The model under review builds one solid part; all positions refer to its coordinate system, in mm. A direction names the side the tool comes from. Coordinates: 2 decimals unless noted, no trailing zeros. Loops run counter-clockwise (first coordinate to the right, second up) from the corner with the lowest first, then second, coordinate; pieces in that order, holes last. Notation, with made-up numbers: M -6.75,14 L 14.25,14 A6 cw 14.25,24 Z; hole C 63.5,-10.5 d6. An arc over 180 degrees is marked long. Write item = value, one per line. Start each with the question number.
Q1. We need section A-A on y = -65.5. Give the boundary of the cut face in (x, z).
Q2. We need section B-B on y = -111. Give the boundary of the cut face in (x, z), and give its area (3 significant figures).
Q3. We need section C-C on z = -3. Count the separate pieces of the cut face and the enclosed holes in it, and give its area (3 significant figures).
Q4. Clearance check with flat-ended pins moving along their axes: pin 1 Ø20 at (y, z) = (-164.5, 1) entering from -X; pin 2 Ø8 at (x, y) = (-12.5, 2.5) entering from +Z; pin 3 Ø5 at (x, y) = (2, -159.5) entering from +Z; pin 4 Ø15 at (x, y) = (-103.97, -30.81) entering from -Z. State where each tip first meets the part, or that it passes through.
Q5. We need section D-D on y = -163. Give the boundary of the cut face in (x, z), and give its area (3 significant figures).
Q6. Wall thickness on probe 1 along Y at (x, z) = (-36, 3.5); probe 2 along Y at (x, z) = (2, 33); probe 3 along Z at (x, y) = (21, -170): over which ranges is each line inside the solid? List them lowest first.
Q7. For faces 1 (the face through (-17.63, 43.38, -5.55)), 2 (the face through (-84.874, 4.13, 0.21)), 3 (the face through (-28.622, -66.375, -9.014)), list the 3-axis set-ups (+Z, -Z, +X, -X, +Y, -Y) from which the entire face can be reached by the end or side of a thin tool; tool diameter is ignored.
Q8. Mouldability with a two-part tool opening along X and no side actions: class faces 4 (the face through (-120.508, -137.418, 0.21)), 5 (the face through (45.486, -200.478, -1.704)), 6 (the face through (-64.24, -171.38, -0.21)) as released by +X, released by -X, zero draft, split by the parting line, or undercut.
from build123d import *

# Parameters (mm, degrees)
BOSS_EXTRUDE1_DEPTH      = 15
BOSS_EXTRUDE1_DEPTH_BACK = 15
SKETCH3_R                = 12.5
SKETCH4_R                = 30
SKETCH4_R_2              = 25
BOSS_EXTRUDE2_DEPTH      = 60
BOSS_EXTRUDE3_DEPTH      = 5
BOSS_EXTRUDE3_DEPTH_BACK = 25
SKETCH5_R                = 30
FILLET1_R                = 10
CUT_EXTRUDE1_START       = -65
SKETCH6_R                = 25
CUT_EXTRUDE1_DEPTH       = 65


with BuildPart() as part:
    # Sketch2 → Revolve1 (revolve)
    with BuildSketch(Plane.XY, mode=Mode.PRIVATE) as revolve1_sk:
        Polygon((0, 47.481515712), (18.484288355, 47.481515712), (18.484288355, 39.394639556), (44.872104392, 39.394639556), (44.872104392, 24.346445364), (35.445928293, 24.346445364), (35.445928293, -47.074965844), (30.007749775, -47.074965844), (30.007749775, -85.142215473), (18.546286043, -160.936690765), (18.546286043, -189.740958038), (45.517560074, -189.740958038), (45.517560074, -202.518484288), (0, -202.518484288), align=None)
    revolve(revolve1_sk.sketch.rotate(Axis((0, 47.481515712, 0), (0, -1, 0)), 180), axis=Axis((0, 47.481515712, 0), (0, -1, 0)))

    # Sketch3 → Boss-Extrude1 (add, two sides: drawn at the far end of the back side and taken through both)
    with BuildSketch(Plane.XY.offset(-BOSS_EXTRUDE1_DEPTH_BACK)):
        Polygon((-42.28533841, 24.346445364), (-86.474429819, 5.279737536), (-86.474429819, -152.790196511), (-42.28533841, -189.740958038), (-42.28533841, -202.518484288), (-44.080740722, -202.518484288), (-121.474429819, -137.802155929), (-121.474429819, 5.226132785), (-42.28533841, 39.394639556), align=None)
        with Locations((-103.974429819, -30.80530006)):
            Circle(SKETCH3_R, mode=Mode.SUBTRACT)
        with Locations((-103.974429819, -115.80530006)):
            Circle(SKETCH3_R, mode=Mode.SUBTRACT)
    extrude(amount=BOSS_EXTRUDE1_DEPTH + BOSS_EXTRUDE1_DEPTH_BACK)

    # Sketch4 → Boss-Extrude2 (add)
    with BuildSketch(Plane(origin=(0, 0, 0), x_dir=(0, 0, -1), z_dir=(1, 0, 0))):
        with Locations(Location((0, -170, 0), (0, 0, 221.149949101))):
            Circle(SKETCH4_R)
        with Locations(Location((0, -170, 0), (0, 0, 141.388518695))):
            Circle(SKETCH4_R_2, mode=Mode.SUBTRACT)
    extrude(amount=BOSS_EXTRUDE2_DEPTH)

    # Sketch5 → Boss-Extrude3 (add, two sides: drawn at the far end of the back side and taken through both)
    with BuildSketch(Plane(origin=(0, 0, 0), x_dir=(0, 0, -1), z_dir=(1, 0, 0)).offset(-BOSS_EXTRUDE3_DEPTH_BACK)):
        with Locations(Location((0, -170, 0), (0, 0, 221.149949101))):
            Circle(SKETCH5_R)
    extrude(amount=BOSS_EXTRUDE3_DEPTH + BOSS_EXTRUDE3_DEPTH_BACK)

    # Fillet1
    # the kernel refuses this fillet: 10 mm, written as the material it adds along each edge
    with BuildSketch(Plane(origin=(-42.974972659, -189.740958038, 15), x_dir=(-1, 0, 0), z_dir=(0, -1, 0))) as fillet1_piece_1_section:
        with BuildLine():
            CenterArc((6.59517437, -10), FILLET1_R, 90, 63.23655504)
            ThreePointArc((-2.333558622, -5.49692026), (-1.076535169, -2.786770672), (0, 0))
            Line((0, 0), (6.59517437, 0))
        make_face()
    fillet1_piece_1 = extrude(amount=12.777526251, mode=Mode.PRIVATE)
    fillet1_piece_1 = split(fillet1_piece_1, bisect_by=Plane(origin=(-48.522573574, -198.80423941, 19.040168561), z_dir=(0.6414797327096047, 0.7671399823518614, 0)), keep=Keep.TOP, mode=Mode.PRIVATE)
    add(fillet1_piece_1)
    with BuildSketch(Plane(origin=(-42.974972659, -189.740958038, -15), x_dir=(0.3907672257300362, 0, -0.9204895302474932), z_dir=(0, -1, 0))) as fillet1_piece_2_section:
        with BuildLine():
            CenterArc((6.627717311, -9.978461215), FILLET1_R, 93.76119811, 63.23655504)
            Line((-2.577177992, -6.070788958), (0, 0))
            ThreePointArc((0, 0), (2.985867888, -0.098039292), (5.971735777, 0))
        make_face()
    fillet1_piece_2 = extrude(amount=12.777526251, mode=Mode.PRIVATE)
    fillet1_piece_2 = split(fillet1_piece_2, bisect_by=Plane(origin=(-48.522573573, -198.80423941, -19.04016856), z_dir=(0.6414797327096047, 0.7671399823518614, 0)), keep=Keep.TOP, mode=Mode.PRIVATE)
    add(fillet1_piece_2)
    with BuildSketch(Plane(origin=(-86.474429819, 5.279737536, 15), x_dir=(0.9181753374265987, 0.39617426688460156, 0), z_dir=(0, 0, -1))) as fillet1_piece_3:
        with BuildLine():
            CenterArc((FILLET1_R * 0.657636628324, FILLET1_R), FILLET1_R, 203.339230224, 66.660769776)
            Line((-FILLET1_R * 0.260538709103, FILLET1_R * 0.603825733115), (0, 0))
            Line((0, 0), (FILLET1_R * 0.657636628324, 0))
        make_face()
    extrude(amount=30)
    with BuildSketch(Plane(origin=(-86.474429819, -152.790196511, 15), x_dir=(0, 1, 0), z_dir=(0, 0, -1))) as fillet1_piece_4:
        with BuildLine():
            CenterArc((FILLET1_R * 0.467346606276, FILLET1_R), FILLET1_R, 219.902248143, 50.097751857)
            Line((-FILLET1_R * 0.299793376076, FILLET1_R * 0.35852026729), (0, 0))
            Line((0, 0), (FILLET1_R * 0.467346606276, 0))
        make_face()
    extrude(amount=30)
    with BuildSketch(Plane(origin=(-42.28533841, -189.740958038, 15), x_dir=(-0.7671399823518606, 0.6414797327096056, 0), z_dir=(0, 0, -1))) as fillet1_piece_5:
        with BuildLine():
            CenterArc((FILLET1_R * 0.363004481318, FILLET1_R), FILLET1_R, 230.097751857, 39.902248143)
            Line((-FILLET1_R * 0.278475251392, FILLET1_R * 0.232860017648), (0, 0))
            Line((0, 0), (FILLET1_R * 0.363004481318, 0))
        make_face()
    extrude(amount=30)
    with BuildSketch(Plane(origin=(-25, -189.740958038, 47.589700656), x_dir=(-1, 0, 0), z_dir=(0, 0, -1))) as fillet1_piece_6_section:
        with BuildLine():
            CenterArc((FILLET1_R, FILLET1_R), FILLET1_R, 180, 90)
            Line((0, FILLET1_R), (0, 0))
            Line((0, 0), (FILLET1_R, 0))
        make_face()
    fillet1_piece_6 = extrude(amount=95.179401313, mode=Mode.PRIVATE)
    fillet1_piece_6 = fillet1_piece_6 & Plane(origin=(-27.186425599, -170, 0), x_dir=(0, -0.6580319345943207, 0.7529900218821333), z_dir=(-1, 0, 0)) * Cylinder(30, 231, mode=Mode.PRIVATE)
    add(fillet1_piece_6)
    # the kernel refuses this fillet: 10 mm, written as the material it takes off along each edge
    with BuildSketch(Plane(origin=(-121.474429819, -137.802155929, 26.683665157), x_dir=(0, 1, 0), z_dir=(0, 0, -1))) as fillet1_2_piece_1:
        with BuildLine():
            CenterArc((FILLET1_R * 0.467346606276, FILLET1_R), FILLET1_R, 219.902248143, 50.097751857)
            Line((-FILLET1_R * 0.299793376076, FILLET1_R * 0.35852026729), (0, 0))
            Line((0, 0), (FILLET1_R * 0.467346606276, 0))
        make_face()
    extrude(amount=53.367330314, mode=Mode.SUBTRACT)
    with BuildSketch(Plane(origin=(-121.474429819, 5.226132785, -31.440915708), x_dir=(0, -1, 0), z_dir=(0, 0, 1))) as fillet1_2_piece_2:
        with BuildLine():
            CenterArc((FILLET1_R * 0.657636628324, FILLET1_R), FILLET1_R, 203.339230224, 66.660769776)
            Line((-FILLET1_R * 0.260538709103, FILLET1_R * 0.603825733115), (0, 0))
            Line((0, 0), (FILLET1_R * 0.657636628324, 0))
        make_face()
    extrude(amount=62.881831416, mode=Mode.SUBTRACT)

    # Sketch6 → Cut-Extrude1 (cut)
    with BuildSketch(Plane(origin=(60, 0, 0), x_dir=(0, 0, -1), z_dir=(1, 0, 0)).offset(CUT_EXTRUDE1_START)):
        with Locations((0, -170)):
            Circle(SKETCH6_R)
    extrude(amount=CUT_EXTRUDE1_DEPTH, mode=Mode.SUBTRACT)


solid = part.part
Returned:
q1.outline = M -121.47,-15 L -86.47,-15 L -86.47,15 L -121.47,15 Z; C 0,0 d60.02
q2.outline = M -121.47,-15 L -115.51,-15 L -115.51,15 L -121.47,15 Z; M -92.43,-15 L -86.47,-15 L -86.47,15 L -92.43,15 Z; C 0,0 d52.2
q2.area = 2,500 mm^2
q3.separate_pieces = 1
q3.enclosed_holes = 3
q3.area = 20,100 mm^2
q4.pin_1 = -101.51
q4.pin_2 = 34.41
q4.pin_3 = 28.91
q4.pin_4 = through
q5.outline = M -91.34,-15 L -74.26,-15 L -74.26,15 L -91.34,15 Z; M -25,-29.17 L 60,-29.17 L 60,-24 L -5,-24 L -5,24 L 60,24 L 60,29.17 L -25,29.17 Z
q5.area = 2,350 mm^2
q6.probe_1 = -202.52 to -189.74, 24.35 to 39.39
q6.probe_2 = -202.52 to -189.74, -47.07 to 39.39
q6.probe_3 = -30 to -25, 25 to 30
q7.face_1 = +Y
q7.face_2 = +Z, -Z
q7.face_3 = none
q8.face_4 = released by -X
q8.face_5 = split by the parting line
q8.face_6 = undercut
